Autodesk Inventor part; units mm, degrees
ref_plane "YZ Plane" through (0, 0, 0) normal (1, 0, 0) x (0, 1, 0)
ref_plane "XZ Plane" through (0, 0, 0) normal (0, 1, 0) x (-1, 0, 0)
ref_plane "XY Plane" through (0, 0, 0) normal (0, 0, 1) x (1, 0, 0)
sketch "스케치1" plane through (0, 0, 0) normal (0, 0, 1) x (1, 0, 0)
  line L0 (33.6127, -21.4008) -> (-33.6127, -21.4008)
  line L1 (-33.6127, -21.4008) -> (-33.6127, 21.4008)
  line L2 (-33.6127, 21.4008) -> (33.6127, 21.4008)
  line L3 (33.6127, 21.4008) -> (33.6127, -21.4008)
  line L4 (33.6127, -21.4008) -> (-33.6127, 21.4008) construction
  line L5 (-33.6127, -21.4008) -> (33.6127, 21.4008) construction
  point P0 (0, 0)
extrude "돌출1" add sketch "스케치1" along normal blind 40
sketch "스케치2" plane through (-33.6127, 21.4008, 0) normal (0, 1, 0) x (1, 0, 0)
  line L0 (67.2253, 0) -> (67.2253, -40)
  line L1 (0, -40) -> (67.2253, -40)
  line L2 (67.2253, -17.9861) -> (27.3679, -17.9861)
  line L3 (27.3679, -17.9861) -> (27.3679, -40)
  line L4 (27.3679, -40) -> (67.2253, -40)
  line L5 (67.2253, -40) -> (67.2253, -17.9861)
  point P0 (33.6127, 0)
extrude "돌출2" cut sketch "스케치2" against normal blind 25
sketch "스케치3" plane through (-6.2447, 21.4008, 17.9861) normal (0, 0, 1) x (1, 0, 0)
  point P0 (6.2447, -21.4008)
sketch "스케치4" plane through (-6.2447, 21.4008, 17.9861) normal (0, 0, 1) x (1, 0, 0)
  point P0 (6.2447, -21.4008)
sketch "스케치5" plane through (-6.2447, 21.4008, 17.9861) normal (0, 0, 1) x (1, 0, 0)
  point P0 (6.2447, -21.4008)
sketch "스케치6" plane through (-33.6127, 21.4008, 0) normal (0, 1, 0) x (1, 0, 0)
  line L0 (27.3679, -17.9861) -> (67.2253, -17.9861)
  line L1 (0, 0) -> (67.2253, 0)
  line L2 (67.2253, -17.9861) -> (39.8016, -17.9861)
  line L3 (39.8016, -17.9861) -> (39.8016, 0)
  line L4 (39.8016, 0) -> (67.2253, 0)
  line L5 (67.2253, 0) -> (67.2253, -17.9861)
  point P0 (33.6127, 0)
sketch "스케치7" plane through (-6.2447, 21.4008, 17.9861) normal (0, 0, 1) x (1, 0, 0)
  line L0 (-27.3679, 0) -> (39.8574, 0)
  line L1 (14.9296, 0) -> (39.8574, -12.2366)
  line L2 (39.8574, 0) -> (39.8574, -42.8017)
  point P0 (6.2447, -21.4008)
extrude "돌출3" cut sketch "스케치7" against normal blind 20
sketch "스케치8" plane through (0, 0, 40) normal (0, 0, 1) x (1, 0, 0)
  point P0 (0, 0)
properties part number "240503_3Dsketch04"
Geometry check sheet. Reference: the model listing, model coordinates, mm. A direction names the side the tool comes from. Round coordinates to 2 decimals unless told otherwise and drop trailing zeros. Order: outer loops, then holes, each group sorted by start corner. A loop starts at its lowest first (then second) coordinate and runs counter-clockwise, first axis right, second up. Notation, with made-up numbers: M 81.5,-28 L 114.5,-28 A10 cw 114.5,-13 Z; hole C -37,-26 d11. An arc over 180 degrees is marked long. Answer in a Markdown table with one row per item.
(1) Sectioned sample at A-A, the plane x = 4. Record the cut outline in (y, z), and give its area (3 significant figures).
Responses:
| item | result |
|---|---|
| outline | M -21.4,0 L 21.4,0 L 21.4,17.99 L -3.6,17.99 L -3.6,40 L -21.4,40 Z |
| area | 1,160 mm² |
(2) Sectioned sample at C-C, the plane z = 5.5. Record the cut outline in (x, y).
Responses:
| item | result |
|---|---|
| outline | M -33.61,-21.4 L 33.61,-21.4 L 33.61,9.16 L 8.68,21.4 L -33.61,21.4 Z |
(3) Tool access check on faces 1 (the face through (-6.245, 9, 29)), 2 (the face through (-33.613, 0, 20)). Record the directions out of +Z, -Z, +X, -X, +Y, -Y that give a thin tool (end or side, any length) a straight path to the whole face; none if there is none.
Responses:
| item | result |
|---|---|
| face 1 | +Z, +X, +Y |
| face 2 | +Z, -Z, -X, +Y, -Y |
(4) Sectioned sample at B-B, the plane z = 36. Record the cut outline in (x, y).
Responses:
| item | result |
|---|---|
| outline | M -33.61,-21.4 L 33.61,-21.4 L 33.61,-3.6 L -6.24,-3.6 L -6.24,21.4 L -33.61,21.4 Z |
(5) Scan lines: probe 1 along X at (y, z) = (1.5, 30); probe 2 along Y at (x, z) = (13, 34); probe 3 along Z at (x, y) = (20, 0). Record each from-to range of solid material in increasing order. Write a range as from..to.
Responses:
| item | result |
|---|---|
| probe 1 | x = -33.61..-6.24 |
| probe 2 | y = -21.4..-3.6 |
| probe 3 | z = 0..17.99 |
(6) Go/stop test with flat-tipped pins: P1, Ø2, axis at y = 13.5, z = 9.5, coming from the +X side; P2, Ø4, axis at x = 7, y = 12, coming from the +Z side; P3, Ø11, axis at x = 8.5, z = 28, coming from the +Y side. Record where each tip stops, or that it passes through.
Responses:
| item | result |
|---|---|
| P1 | stops at x = 26.82 |
| P2 | stops at z = 17.99 |
| P3 | stops at y = -3.6 |
